from build123d import *

# Parameters (mm, degrees)
EXTRUDE_1_DEPTH     = 30
SKETCH_3_W          = 24
SKETCH_3_H          = 35.230133155
CUT_EXTRUDE_1_DEPTH = 33
CUT_EXTRUDE_2_DEPTH = 5


with BuildPart() as part:
    # 草图1 → 凸台-拉伸1 (new body)
    with BuildSketch(Plane.XY):
        Polygon((16.339285714, 24.209821429), (9.839285714, 24.209821429), (9.839285714, 17.209821429), (-13.660714286, -6.290178571), (-20.660714286, -6.290178571), (-20.660714286, -12.790178571), (16.339285714, -12.790178571), align=None)
    extrude(amount=EXTRUDE_1_DEPTH)

    # 草图3 → 切除-拉伸1 (cut)
    with BuildSketch(Plane.ZY.offset(20.660714286)):
        with Locations((15, 8.824888007)):
            Rectangle(SKETCH_3_W, SKETCH_3_H)
    extrude(amount=-CUT_EXTRUDE_1_DEPTH, mode=Mode.SUBTRACT)

    # 草图4 → 切除-拉伸2 (cut, through all)
    with BuildSketch(Plane(origin=(0, -8.790178571, 0), x_dir=(1, 0, 0), z_dir=(0, 1, 0))):
        with BuildLine():
            Line((-9.160714286, -10.75), (0.339285714, -10.75))
            ThreePointArc((0.339285714, -10.75), (4.589285714, -15), (0.339285714, -19.25))
            Line((0.339285714, -19.25), (-9.160714286, -19.25))
            ThreePointArc((-9.160714286, -19.25), (-13.410714286, -15), (-9.160714286, -10.75))
        make_face()
    cut_extrude_2 = extrude(amount=-CUT_EXTRUDE_2_DEPTH, mode=Mode.SUBTRACT)

    # 镜向1: 切除-拉伸2 across plane
    add(cut_extrude_2.mirror(Plane(origin=(1.774553571, 1.774553571, 0), x_dir=(0, 0, 1), z_dir=(0.707106781, 0.707106781, 0))), mode=Mode.SUBTRACT)


solid = part.part
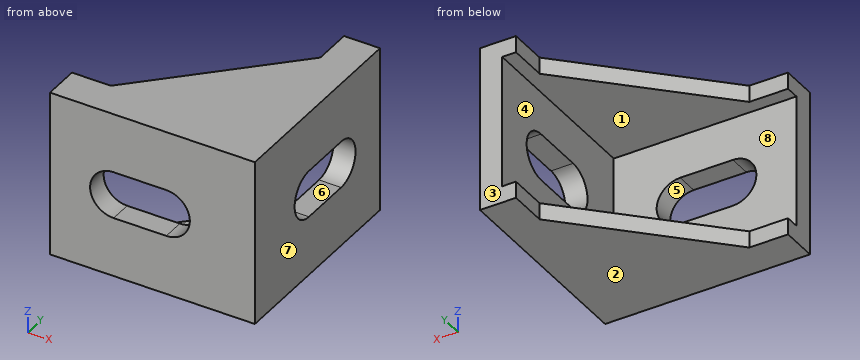
Build history of the part. All positions in model axes, mm. Face numbers are marked on the shaded views. A direction names the side the tool comes from. Round coordinates to 2 decimals unless told otherwise and drop trailing zeros. Loops run counter-clockwise (first coordinate to the right, second up) from the corner with the lowest first, then second, coordinate; pieces in that order, holes last. Notation, with made-up numbers: (-28, -11) -> (-7, -11) arc R29 cw to (-7, 26) -> close; hole circle Ø9 at (48, -28.75). An arc over 180 degrees is marked (long way). One line per item, written item: value. Start each with the question number.
Q1. Cut at D-D on z = 26.25. List the corners of the cut face in (x, y), plus the area to 3 significant figures.
Q2. Probe line 1 along Z through (x, y) = (2, -4); line 2 along Y through (x, z) = (-9, 6.75); line 3 along X through (y, z) = (-7, 25.5). List the from-to ranges inside material, lowest first.
Q3. Two-plate mould, pull along Z, no slides. Class the marked faces 1, 2, 3 and 4: released by +Z, released by -Z, zero draft, split by the parting line, or undercut.
Q4. Cut at B-B on y = 16. List the corners of the cut face in (x, z).
Q5. Cut at C-C on x = 4. List the corners of the cut face in (y, z).
Q6. Drop flat-ended pins along their axis: pin 1 Ø6 at (x, z) = (2, 17.5) entering from +Y; pin 2 Ø4.5 at (x, y) = (-3, -10.5) entering from -Z; pin 3 Ø2.5 at (y, z) = (19.5, 1) entering from -X; pin 4 Ø2 at (y, z) = (2, 19) entering from -X. Give the stop position or say it passes through.
Q7. 3-axis set-ups, long thin cutter, end or side, ignore diameter. For the marked faces 5, 6, 7 and 8: which of +Z, -Z, +X, -X, +Y, -Y reach the whole face in a straight line?
Q8. Cut at A-A on z = 15. List the corners of the cut face in (x, y).
Computed:
1. outline: (-20.66, -12.79) -> (16.34, -12.79) -> (16.34, 24.21) -> (12.34, 24.21) -> (12.34, -8.79) -> (-20.66, -8.79) -> close
1. area: 280 mm²
2. line 1: 0 to 3, 27 to 30
2. line 2: -12.79 to -8.79
2. line 3: 12.34 to 16.34
3. face 1: undercut
3. face 2: released by -Z
3. face 3: zero draft
3. face 4: undercut
4. outline: (8.63, 0) -> (16.34, 0) -> (16.34, 12.31) -> (12.34, 12.31) -> (12.34, 3) -> (8.63, 3) -> close; (8.63, 27) -> (12.34, 27) -> (12.34, 17.69) -> (16.34, 17.69) -> (16.34, 30) -> (8.63, 30) -> close
5. outline: (-12.79, 0) -> (11.37, 0) -> (11.37, 3) -> (-8.79, 3) -> (-8.79, 12.84) -> (-12.79, 12.84) -> close; (-12.79, 17.16) -> (-8.79, 17.16) -> (-8.79, 27) -> (11.37, 27) -> (11.37, 30) -> (-12.79, 30) -> close
6. pin 1: y = -8.79
6. pin 2: z = 0
6. pin 3: x = 9.84
6. pin 4: x = 12.34
7. face 5: +Y, -Y
7. face 6: +X, -X
7. face 7: +Z, -Z, +X, +Y, -Y
7. face 8: -X, +Y
8. outline: (-20.66, -12.79) -> (-13.41, -12.79) -> (-13.41, -8.79) -> (-20.66, -8.79) -> close; (4.59, -12.79) -> (16.34, -12.79) -> (16.34, -1.04) -> (12.34, -1.04) -> (12.34, -8.79) -> (4.59, -8.79) -> close; (12.34, 16.96) -> (16.34, 16.96) -> (16.34, 24.21) -> (12.34, 24.21) -> close
